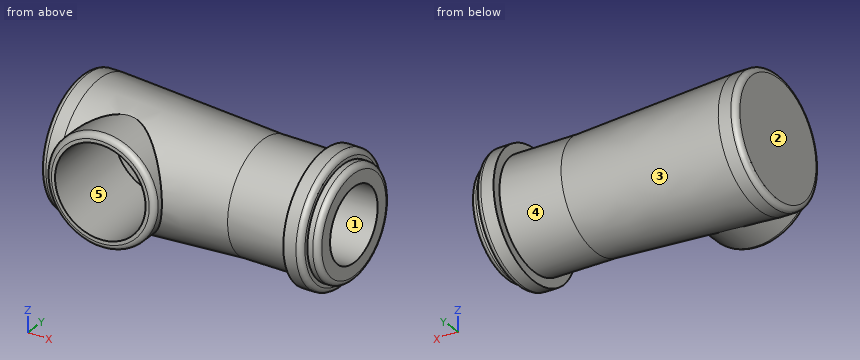
```python
from build123d import *

# Parameters (mm, degrees)
F2_R     = 15
F3_DEPTH = 19
F4_R     = 12.5
F5_DEPTH = 25
F6_R     = 1.5
F7_R     = 1.5


with BuildPart() as f1:
    # F0 (on Front) → F1 (revolve)
    with BuildSketch(Plane.XZ):
        Polygon((0, 17.5), (0, 0), (60, 0), (60, 10), (75, 10), (75, 15), (72, 15), (72, 17.5), (67, 17.5), (67, 15), (50, 15), (5, 17.5), align=None)
    revolve(axis=Axis((30, 0, 0), (1, 0, 0)))

    # F2 (on Front) → F3 (join)
    with BuildSketch(Plane.XZ):
        with Locations((17.5, 0)):
            Circle(F2_R)
    extrude(amount=F3_DEPTH)

    # F4 (on face) → F5 (cut)
    with BuildSketch(Plane.XZ.offset(19)):
        with Locations((17.5, 0)):
            Circle(F4_R)
    extrude(amount=-F5_DEPTH, mode=Mode.SUBTRACT)

    # F6
    f6_edges = [f1.edges().sort_by_distance(p)[0] for p in [
        (72, 0, -17.5),
        (75, 0, -15),
        (0, 0, -17.5),
    ]]
    fillet(f6_edges, radius=F6_R)

    # F7
    f7_edges = [f1.edges().sort_by_distance(p)[0] for p in [
        (2.5, -19, 0),
    ]]
    fillet(f7_edges, radius=F7_R)


solid = f1.part
```
The listing builds one solid part. Answer for the finished solid, in the listing's coordinates (mm). Face numbers are marked on the shaded views. A direction names the side the tool comes from. Coordinates: 2 decimals unless noted, no trailing zeros. Write each loop counter-clockwise with the first axis right and the second up, starting at its lowest first coordinate (ties: lowest second). Pieces come first, ordered by that corner, then holes. Notation, with made-up numbers: M -38.5,39 L -21.5,39 A11 cw -21.5,49 Z; hole C 72,40 d6. An arc over 180 degrees is marked long. Use a Markdown table: item, result. Add a question column.
1. Straight lines are drawn through the part: line 1 along Y through (x, z) = (65.75, 0); line 2 along Z through (x, y) = (22, -4). For each, find the intervals that lie inside material, in ascending order. Write a range as [from, to].
2. Which of the six approach directions +Z, -Z, +X, -X, +Y, -Y give full straight-line access (tool end or side, diameter ignored) to the marked faces 4 and 5?
3. Given P1, Ø9.5, axis at y = -0.5, z = 1.5, coming from the +X side; P2, Ø8, axis at x = 16, z = 1.5, coming from the -Y side; P3, Ø12, axis at x = 34, y = -1, coming from the +Z side, each flat-ended and moving along its own axis, determine where each tip first touches the part or whether it passes through.
4. Section C-C (x = 43) is taken. Give the vertices of the cut face in (y, z), plus the area to 3 significant figures.
5. Section A-A (y = 0) is taken. Give the vertices of the cut face in (x, z), plus the area to 3 significant figures.
6. Section B-B (x = 17.5) is taken. Give the vertices of the cut face in (y, z), plus the area to 3 significant figures.
7. For a pull along Y with two mould halves and no side action, classify the marked faces 1, 2 and 3 as +Y half, -Y half, draft (parallel to the pull), parting line (faces both ways), or undercut.
Data:
| question | item | result |
|---|---|---|
| 1 | line 1 | y = [-15, -10], [10, 15] |
| 1 | line 2 | z = [-16.07, -11.66], [11.66, 16.07] |
| 2 | face 4 | none |
| 2 | face 5 | -Y |
| 3 | P1 | stops at x = 60 |
| 3 | P2 | stops at y = 6 |
| 3 | P3 | stops at z = 16.22 |
| 4 | outline | C 0,0 d30.78 |
| 4 | area | 744 mm2 |
| 5 | outline | M 0,-16 A1.5 ccw 1.5,-17.5 L 5,-17.5 L 50,-15 L 67,-15 L 67,-17.5 L 70.5,-17.5 A1.5 ccw 72,-16 L 72,-15 L 73.5,-15 A1.5 ccw 75,-13.5 L 75,-10 L 60,-10 L 60,10 L 75,10 L 75,13.5 A1.5 ccw 73.5,15 L 72,15 L 72,16 A1.5 ccw 70.5,17.5 L 67,17.5 L 67,15 L 50,15 L 5,17.5 L 1.5,17.5 A1.5 ccw 0,16 Z; hole C 17.5,0 d25 |
| 5 | area | 1,620 mm2 |
| 6 | outline | M -19,-13.5 A1.5 ccw -17.5,-15 L -7.58,-15 A16.81 ccw long -7.58,15 L -17.5,15 A1.5 ccw -19,13.5 L -19,12.5 L 6,12.5 L 6,-12.5 L -19,-12.5 Z |
| 6 | area | 406 mm2 |
| 7 | face 1 | undercut |
| 7 | face 2 | draft |
| 7 | face 3 | parting line |
